Source: CAD feature listing. Evaluate the final solid. Frame: model axes, mm. Face numbers are marked on the shaded views. A direction names the side the tool comes from. Give positions to 0.01 mm unless a question says otherwise; leave off trailing zeros. Write each loop counter-clockwise with the first axis right and the second up, starting at its lowest first coordinate (ties: lowest second). Pieces come first, ordered by that corner, then holes. Notation, with made-up numbers: M 38.5,59 L 87.5,59 A22 cw 87.5,91 Z; hole C 43,55 d8. An arc over 180 degrees is marked long. Return JSON: item names as keys, results as strings.
```python
from build123d import *

# Parameters (mm, degrees)
SKETCH11_W          = 35.56
SKETCH11_H          = 32.385
SKETCH11_R          = 2.032
BOSS_EXTRUDE1_DEPTH = 6.35
SKETCH14_W          = 35.56
SKETCH14_H          = 3.302
BOSS_EXTRUDE2_DEPTH = 28.702
CUT_EXTRUDE1_REACH  = 50.853
SKETCH15_R          = 9.017
SKETCH16_W          = 35.56
SKETCH16_H          = 15.113
CUT_EXTRUDE2_DEPTH  = 57.009879745


with BuildPart() as part:
    # Sketch11 → Boss-Extrude1 (new body)
    with BuildSketch(Plane(origin=(0, 0, 0), x_dir=(1, 0, 0), z_dir=(0, 1, 0))):
        with Locations((17.78, 16.1925)):
            Rectangle(SKETCH11_W, SKETCH11_H)
        with Locations(Location((5.08, 27.6225, 0), (0, 0, 270))):
            Circle(SKETCH11_R, mode=Mode.SUBTRACT)
        with Locations(Location((30.48, 27.6225, 0), (0, 0, 270))):
            Circle(SKETCH11_R, mode=Mode.SUBTRACT)
        with Locations(Location((17.78, 6.7945, 0), (0, 0, 270))):
            Circle(SKETCH11_R, mode=Mode.SUBTRACT)
    extrude(amount=BOSS_EXTRUDE1_DEPTH)

    # Sketch14 → Boss-Extrude2 (add)
    with BuildSketch(Plane.XZ):
        with Locations((17.78, -16.764)):
            Rectangle(SKETCH14_W, SKETCH14_H)
    extrude(amount=BOSS_EXTRUDE2_DEPTH)

    # Sketch15 → Cut-Extrude1 (cut, up to next)
    with BuildSketch(Plane.XY.offset(-15.113), mode=Mode.PRIVATE) as cut_extrude1_sk1:
        with Locations((17.78, -15.748)):
            Circle(SKETCH15_R)
    cut_extrude1_tool1 = extrude(cut_extrude1_sk1.sketch, amount=-CUT_EXTRUDE1_REACH, mode=Mode.PRIVATE) & part.part
    add(cut_extrude1_tool1.solids().sort_by_distance((17.78, -15.748, -15.113))[0], mode=Mode.SUBTRACT)

    # Sketch16 → Cut-Extrude2 (cut, through all)
    with BuildSketch(Plane.XZ):
        with Locations((17.78, -7.5565)):
            Rectangle(SKETCH16_W, SKETCH16_H)
    extrude(amount=-CUT_EXTRUDE2_DEPTH, mode=Mode.SUBTRACT)


solid = part.part
```
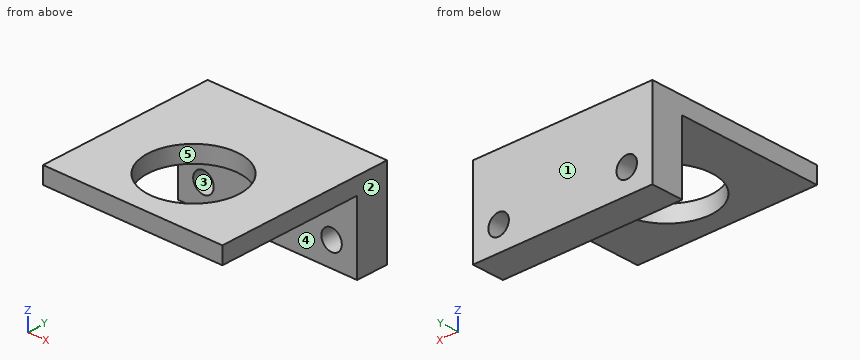
1) Cut plane D-D, the plane z = -27.5. Return the cut outline in (x, y).
Numbers:
{"outline": "M 0,0 L 3.05,0 L 3.05,6.35 L 0,6.35 Z; M 7.11,0 L 28.45,0 L 28.45,6.35 L 7.11,6.35 Z; M 32.51,0 L 35.56,0 L 35.56,6.35 L 32.51,6.35 Z"}
2) Contact query for a flat-ended pin moving along its axis: pin 1 Ø4 at (x, y) = (31, -18.5) entering from -Z (3 decimals). Output: stop coordinate, or through.
Numbers:
{"pin 1": "stops at z = -18.415"}
3) Cut plane B-B, the plane y = -23.5. Return the cut outline in (x, z) (3 decimals).
Numbers:
{"outline": "M 0,-18.415 L 13.174,-18.415 L 13.174,-15.113 L 0,-15.113 Z; M 22.386,-18.415 L 35.56,-18.415 L 35.56,-15.113 L 22.386,-15.113 Z"}
4) Cut plane C-C, the plane x = 8. Return the cut outline in (y, z) (3 decimals), then the cut area to 3 significant figures.
Numbers:
{"outline": "M -28.702,-18.415 L 0,-18.415 L 0,-32.385 L 6.35,-32.385 L 6.35,-15.113 L -28.702,-15.113 Z", "area": "204 mm²"}
5) Line query: line 1 (Z direction, x = 5, y = 3) (3 decimals); line 2 (Y direction, x = 34.5, z = -19.5); line 3 (Z direction, x = 4, y = -7.5) (3 decimals). Output: solid intervals per line, ascending. Write a range as [from, to].
Numbers:
{"line 1": "z = [-32.385, -29.653], [-25.592, -15.113]", "line 2": "y = [0, 6.35]", "line 3": "z = [-18.415, -15.113]"}
6) Set-up query: the marked faces 4 and 5. Return all of +Z, -Z, +X, -X, +Y, -Y with unobstructed straight access to the full face (end or side cutting, diameter ignored); none if empty.
Numbers:
{"face 4": "-Z, +X, -X, -Y", "face 5": "+Z, -Z"}
7) Draft query along X for the marked faces 1, 2 and 3. Return one class per face: released by +X, released by -X, zero draft, split by the parting line, or undercut.
Numbers:
{"face 1": "zero draft", "face 2": "released by +X", "face 3": "undercut"}
8) Cut plane A-A, the plane x = 17.78. Return the cut outline in (y, z) (3 decimals).
Numbers:
{"outline": "M -28.702,-18.415 L -24.765,-18.415 L -24.765,-15.113 L -28.702,-15.113 Z; M -6.731,-18.415 L 0,-18.415 L 0,-32.385 L 6.35,-32.385 L 6.35,-15.113 L -6.731,-15.113 Z"}
